Work out the finished part from the listing and answer in its coordinate system (mm). Face numbers are marked on the shaded views. A direction names the side the tool comes from. Give positions to 0.01 mm unless a question says otherwise; leave off trailing zeros. Order: outer loops, then holes, each group sorted by start corner. A loop starts at its lowest first (then second) coordinate and runs counter-clockwise, first axis right, second up. Notation, with made-up numbers: (-9, 23) - (15, 23) arc R25 ccw to (15, 55) - close; hole circle Ø7 at (-38, 8). An arc over 180 degrees is marked (long way). Put each result on its own line as item: value.
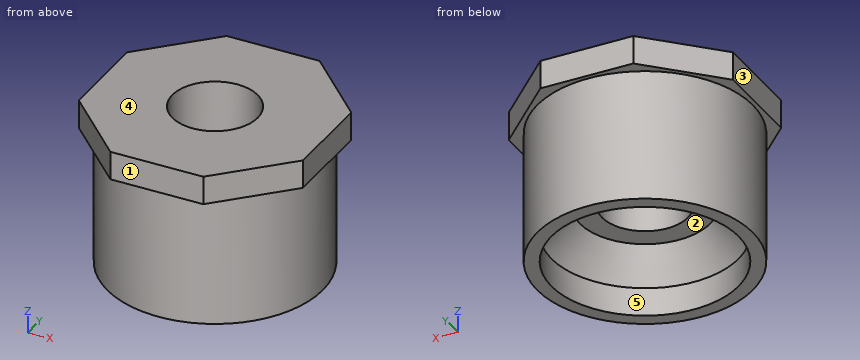
```python
from build123d import *

# Parameters (mm, degrees)
F0_R     = 9.525
F1_DEPTH = 6.35
F2_R     = 24.030165
F2_R_2   = 9.525
F3_DEPTH = 29.464
F4_R     = 20.855165
F5_DEPTH = 12.7
F6_SIZE  = 6.35


with BuildPart() as f1:
    # F0 (on Top) → F1 (new body)
    with BuildSketch(Plane.XY):
        Polygon((-10.355339, -25), (10.355339, -25), (25, -10.355339), (25, 10.355339), (10.355339, 25), (-10.355339, 25), (-25, 10.355339), (-25, -10.355339), align=None)
        Circle(F0_R, mode=Mode.SUBTRACT)
    extrude(amount=F1_DEPTH)

    # F2 (on face) → F3 (join)
    with BuildSketch(Plane(origin=(0, 0, 0), x_dir=(1, 0, 0), z_dir=(0, 0, -1))):
        Circle(F2_R)
        Circle(F2_R_2, mode=Mode.SUBTRACT)
    extrude(amount=F3_DEPTH)

    # F4 (on face) → F5 (cut)
    with BuildSketch(Plane(origin=(0, 0, -29.464), x_dir=(1, 0, 0), z_dir=(0, 0, -1))):
        Circle(F4_R)
    extrude(amount=-F5_DEPTH, mode=Mode.SUBTRACT)

    # F6
    f6_edges = [f1.edges().sort_by_distance(p)[0] for p in [
        (-20.855165, 0, -16.764),
    ]]
    chamfer(f6_edges, length=F6_SIZE)


solid = f1.part
```
(1) Straight lines are drawn through the part: line 1 (Y direction, x = 0, z = -27.5); line 2 (Y direction, x = 0, z = -11.75) (3 decimals). For each, find the intervals that lie inside material, in ascending order.
Geometry check:
line 1: y = -24.03 to -20.86, 20.86 to 24.03
line 2: y = -24.03 to -9.525, 9.525 to 24.03
(2) Section A-A, the plane y = 0 is taken. Write down the section's boundary in (x, z) (3 decimals), then the cut area to 3 significant figures.
Geometry check:
outline: (-25, 0) - (-24.03, 0) - (-24.03, -29.464) - (-20.855, -29.464) - (-20.855, -23.114) - (-14.505, -16.764) - (-9.525, -16.764) - (-9.525, 6.35) - (-25, 6.35) - close; (9.525, -16.764) - (14.505, -16.764) - (20.855, -23.114) - (20.855, -29.464) - (24.03, -29.464) - (24.03, 0) - (25, 0) - (25, 6.35) - (9.525, 6.35) - close
area: 804 mm²
(3) Section D-D, the plane z = -24.5 is taken. Write down the section's boundary in (x, y), then the cut area to 3 significant figures.
Geometry check:
outline: circle Ø48.06 at (0, 0); hole circle Ø41.71 at (0, 0)
area: 448 mm²
(4) Section C-C, the plane z = -12.5 is taken. Write down the section's boundary in (x, y) (3 decimals).
Geometry check:
outline: circle Ø48.06 at (0, 0); hole circle Ø19.05 at (0, 0)
(5) Given pin 1 (1.5 mm diameter, centred on y = 16.5, z = 0.5, fed in from +X); pin 2 (14.5 mm diameter, centred on x = -4.5, y = 3, fed in from -Z); pin 3 (5 mm diameter, centred on x = -6.5, z = -8.5, fed in from -Y), each flat-ended and moving along its own axis, determine where each tip first touches the part or whether it passes through.
Geometry check:
pin 1: stops at x = 19.61
pin 2: stops at z = -16.76
pin 3: stops at y = -23.69
(6) Determine the mould class of the marked faces 3, 4 and 5 for opening direction X: pulls with the +X half, pulls with the -X half, needs draft (parallel to the pull), parting line crosses it, or undercut.
Geometry check:
face 3: pulls with the -X half
face 4: needs draft
face 5: undercut
(7) A tool of negligible diameter and unlimited length cuts with its end or side. For the marked faces 1 and 2, from which of +Z, -Z, +X, -X, +Y, -Y can it reach the whole face along a straight path? Write none if from no direction.
Geometry check:
face 1: +Z, -Z, +X, -X, -Y
face 2: -Z
